```python
from build123d import *

# Parameters (mm, degrees)
SKETCH4_R           = 26.67
SKETCH4_R_2         = 3.175
SKETCH4_R_3         = 4
BOSS_EXTRUDE1_DEPTH = 6.35


with BuildPart() as part:
    # Sketch4 → Boss-Extrude1 (new body)
    with BuildSketch(Plane.XY):
        with BuildLine():
            Line((-112.821947343, -67.861519054), (-0.515655425, 42.221127865))
            ThreePointArc((-0.515655425, 42.221127865), (5.060574998, 45.411581565), (11.484788098, 45.464747253))
            ThreePointArc((11.484788098, 45.464747253), (34.621914338, 31.626992395), (46.315565637, 7.335664942))
            ThreePointArc((46.315565637, 7.335664942), (46.8988099, 5.456870428), (47.991424982, 3.820950204))
            Line((47.991424982, 3.820950204), (112.830192448, -68.228316343))
            ThreePointArc((112.830192448, -68.228316343), (113.646801884, -83.357459106), (99.032580967, -87.355253332))
            Line((99.032580967, -87.355253332), (7.333742713, -47.300802353))
            ThreePointArc((7.333742713, -47.300802353), (5.650340933, -46.801981002), (3.896034016, -46.730766304))
            ThreePointArc((3.896034016, -46.730766304), (-2.51262623, -46.825530534), (-8.874346459, -46.045516343))
            ThreePointArc((-8.874346459, -46.045516343), (-11.116219354, -45.973658852), (-13.268973959, -46.603583598))
            Line((-13.268973959, -46.603583598), (-99.204524399, -87.377892758))
            ThreePointArc((-99.204524399, -87.377892758), (-114.270940187, -83.381465438), (-112.821947343, -67.861519054))
        make_face()
        Circle(SKETCH4_R, mode=Mode.SUBTRACT)
        with Locations((103.862003689, -76.298992609)):
            Circle(SKETCH4_R_2, mode=Mode.SUBTRACT)
        with Locations((-104.376429258, -76.477634727)):
            Circle(SKETCH4_R_2, mode=Mode.SUBTRACT)
        with Locations((-10.093942759, -37.671107225)):
            Circle(SKETCH4_R_3, mode=Mode.SUBTRACT)
        with Locations((-31.946929727, -22.369481018)):
            Circle(SKETCH4_R_3, mode=Mode.SUBTRACT)
        with Locations((27.577164466, -27.577164466)):
            Circle(SKETCH4_R_3, mode=Mode.SUBTRACT)
        with Locations((37.671107225, 10.093942759)):
            Circle(SKETCH4_R_3, mode=Mode.SUBTRACT)
        with Locations((22.369481018, 31.946929727)):
            Circle(SKETCH4_R_3, mode=Mode.SUBTRACT)
        with BuildLine():
            Line((-86.689084945, -55.583778017), (-55.691219904, -25.199665298))
            ThreePointArc((-55.691219904, -25.199665298), (-50.133633158, -23.190261002), (-44.975951587, -26.075186805))
            Line((-44.975951587, -26.075186805), (-36.452805068, -37.70754969))
            ThreePointArc((-36.452805068, -37.70754969), (-35.294757483, -43.654797982), (-39.140960913, -48.336416892))
            Line((-39.140960913, -48.336416892), (-78.661972473, -67.088166726))
            ThreePointArc((-78.661972473, -67.088166726), (-87.543228095, -64.73237799), (-86.689084945, -55.583778017))
        make_face(mode=Mode.SUBTRACT)
        with BuildLine():
            Line((34.66659199, -39.378036032), (47.195108172, -22.323593379))
            ThreePointArc((47.195108172, -22.323593379), (52.574176498, -19.430906367), (58.213255891, -21.776710666))
            Line((58.213255891, -21.776710666), (91.616099201, -58.894170716))
            ThreePointArc((91.616099201, -58.894170716), (92.097468974, -67.812402239), (83.482770328, -70.16899673))
            Line((83.482770328, -70.16899673), (37.551410836, -50.105979333))
            ThreePointArc((37.551410836, -50.105979333), (33.530211234, -45.435462365), (34.66659199, -39.378036032))
        make_face(mode=Mode.SUBTRACT)
    extrude(amount=BOSS_EXTRUDE1_DEPTH)


solid = part.part
```
For this review, take the finished solid that the model builds, in its own axes (mm). A direction names the side the tool comes from. Round coordinates to 2 decimals unless told otherwise and drop trailing zeros. Write each loop counter-clockwise with the first axis right and the second up, starting at its lowest first coordinate (ties: lowest second). Pieces come first, ordered by that corner, then holes. Notation, with made-up numbers: (-38.5, 43) -> (-12.5, 43) arc R28 cw to (-12.5, 68) -> close; hole circle Ø9 at (64.5, 30). An arc over 180 degrees is marked (long way). Use one line per item in the form item = value.
Q1. To check wall thickness, follow probe 1 along X at (y, z) = (11.5, 4); probe 2 along X at (y, z) = (-35.5, 2.5); probe 3 along X at (y, z) = (-57.5, 0.75). State the ranges of each line that lie inside material, in increasing order. Write a range as from..to.
Resolved:
probe_1 = -31.86..-24.06, 24.06..33.93, 41.42..45.46
probe_2 = -79.81..-66.2, -38.07..-13.45, -6.73..37.52, 70.56..83.38
probe_3 = -102.25..-88.08, -58.45..-36.23, 30.68..54.48, 90.36..103.18
Q2. Machinability: for faces 1 (the flat face through (53.83, -67.61, 3.13)), 2 (the cylindrical face through (4.973, 45.388, 3.131)), 3 (the flat face through (40.843, -30.97, 3.131)), which of the approach directions +Z, -Z, +X, -X, +Y, -Y give a long, thin tool a straight path to every point of the face, cutting with its end or side? Answer none if there is none.
Resolved:
face_1 = +Z, -Z, -Y
face_2 = +Z, -Z, +Y
face_3 = +Z, -Z
Q3. Consider section C-C (y = -64). State the section outline as (x, z) points.
Resolved:
outline = (-108.88, 0) -> (-87.99, 0) -> (-87.99, 6.35) -> (-108.88, 6.35) -> close; (-72.15, 0) -> (-49.93, 0) -> (-49.93, 6.35) -> (-72.15, 6.35) -> close; (45.56, 0) -> (69.36, 0) -> (69.36, 6.35) -> (45.56, 6.35) -> close; (93.43, 0) -> (109.03, 0) -> (109.03, 6.35) -> (93.43, 6.35) -> close
Q4. The part is to be moulded in two halves that separate along X. For faces 4 (the flat face through (79.96, -31.7, 3.13)), 5 (the flat face through (-57.455, -13.591, 3.131)), 6 (the flat face through (74.681, -40.076, 3.131)), say which applies: released by +X, released by -X, zero draft, split by the parting line, or undercut.
Resolved:
face_4 = released by +X
face_5 = released by -X
face_6 = undercut
Q5. Clearance check with flat-ended pins moving along their axes: pin 1 Ø1 at (x, z) = (-69.5, 5.5) entering from +Y; pin 2 Ø7 at (x, y) = (-10.09, -37.67) entering from -Z. State where each tip first meets the part, or that it passes through.
Resolved:
pin_1 = -24.91
pin_2 = through
Q6. Consider section B-B (z = 1). State how many separate pieces and enclosed holes the cut face has, then the cut area to 3 significant figures.
Resolved:
separate_pieces = 1
enclosed_holes = 10
area = 8,300 mm²
Q7. Consider section A-A (y = 0). State the section outline as (x, z) points, then the cut area to 3 significant figures.
Resolved:
outline = (-43.59, 0) -> (-26.67, 0) -> (-26.67, 6.35) -> (-43.59, 6.35) -> close; (26.67, 0) -> (51.43, 0) -> (51.43, 6.35) -> (26.67, 6.35) -> close
area = 265 mm²
